Read the model definition and answer for the solid it produces. Units are mm, in the model's axes. Coordinates: 2 decimals unless noted, no trailing zeros. Write each loop counter-clockwise with the first axis right and the second up, starting at its lowest first coordinate (ties: lowest second). Pieces come first, ordered by that corner, then holes.
(1) Section B-B on x = 129.5 is taken. Write down the section's boundary in (y, z), then the cut area to 3 significant figures.
(2) Section C-C on y = 25 is taken. Write down the section's boundary in (x, z), then the cut area to 3 significant figures.
(3) Section A-A on z = -8.5 is taken. Write down the section's boundary in (x, y).
(4) Find the intervals of material crossed by probe 1 along Y at (x, z) = (197.5, -18.1); probe 2 along Y at (x, z) = (151, -8); probe 3 along Y at (x, z) = (14, -14.5), in increasing order.
(5) Given pin 1 (4.5 mm diameter, centred on y = 92.5, z = -13.5, fed in from -X); pin 2 (3 mm diameter, centred on x = 98, z = -13, fed in from +Y); pin 3 (2.5 mm diameter, centred on x = 197.5, y = 80, fed in from -Z), each flat-ended and moving along its own axis, determine where each tip first touches the part or whether it passes through.
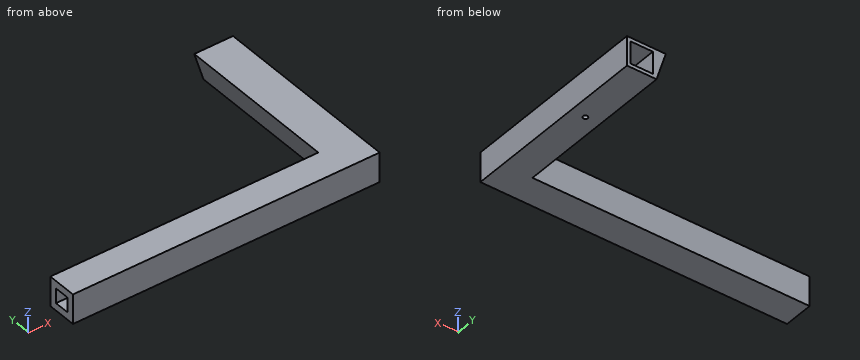
from build123d import *

# Parameters (mm, degrees)
ESQUISSE1_W             = 207.5
ESQUISSE1_H             = 20
BOSS_EXTRU_1_DEPTH      = 20
BOSS_EXTRU_2_DEPTH      = 110
ESQUISSE3_W             = 10
ESQUISSE3_H             = 10
ENL_V_MAT_EXTRU_1_DEPTH = 30
D_GAGEMENT_M31_D        = 3.2
D_GAGEMENT_M31_DEPTH    = 10
D_GAGEMENT_M31_TIP      = 0.96137699
ESQUISSE6_W             = 15
ESQUISSE6_H             = 15
ENL_V_MAT_EXTRU_2_DEPTH = 60


with BuildPart() as part:
    # Esquisse1 → Boss.-Extru.1 (new body)
    with BuildSketch(Plane(origin=(0, 0, 0), x_dir=(1, 0, 0), z_dir=(0, 1, 0))):
        with Locations((103.75, 10)):
            Rectangle(ESQUISSE1_W, ESQUISSE1_H)
    extrude(amount=BOSS_EXTRU_1_DEPTH)

    # Esquisse2 → Boss.-Extru.2 (add)
    with BuildSketch(Plane(origin=(0, 20, 0), x_dir=(1, 0, 0), z_dir=(0, 1, 0))):
        Polygon((207.5, 20), (187.5, 20), (181.270693681, 0), (207.5, 0), align=None)
    extrude(amount=BOSS_EXTRU_2_DEPTH)

    # Esquisse3 → Enlèv. mat.-Extru.1 (cut)
    with BuildSketch(Plane.ZY):
        with Locations((-10, 10)):
            Rectangle(ESQUISSE3_W, ESQUISSE3_H)
    extrude(amount=-ENL_V_MAT_EXTRU_1_DEPTH, mode=Mode.SUBTRACT)

    # Dégagement M31
    with Locations(Plane(origin=(0, 0, -20), x_dir=(-1, 0, 0), z_dir=(0, 0, -1))):
        with Locations((-197.5, 80)):
            Hole(D_GAGEMENT_M31_D / 2, depth=D_GAGEMENT_M31_DEPTH)
            with Locations((0, 0, -(D_GAGEMENT_M31_DEPTH + D_GAGEMENT_M31_TIP / 2))):  # 118° drill point
                Cone(0, D_GAGEMENT_M31_D / 2, D_GAGEMENT_M31_TIP, mode=Mode.SUBTRACT)

    # Esquisse6 → Enlèv. mat.-Extru.2 (cut)
    with BuildSketch(Plane(origin=(0, 130, 0), x_dir=(1, 0, 0), z_dir=(0, 1, 0))):
        with Locations((197.5, 10)):
            Rectangle(ESQUISSE6_W, ESQUISSE6_H)
    extrude(amount=-ENL_V_MAT_EXTRU_2_DEPTH, mode=Mode.SUBTRACT)


solid = part.part
Response:
1. outline: (0, -20) - (20, -20) - (20, 0) - (0, 0) - close
1. area: 400 mm2
2. outline: (181.27, 0) - (187.5, -20) - (207.5, -20) - (207.5, 0) - close
2. area: 462 mm2
3. outline: (0, 0) - (207.5, 0) - (207.5, 130) - (205, 130) - (205, 70) - (190, 70) - (190, 130) - (183.92, 130) - (183.92, 20) - (0, 20) - (0, 15) - (30, 15) - (30, 5) - (0, 5) - close
4. probe 1: y = 0 to 78.4, 81.6 to 130
4. probe 2: y = 0 to 20
4. probe 3: y = 0 to 5, 15 to 20
5. pin 1: stops at x = 184.77
5. pin 2: stops at y = 20
5. pin 3: stops at z = -2.5
